from build123d import *

# Parameters (mm, degrees)
SKETCH_1_W      = 50
SKETCH_1_H      = 50
EXTRUDE_1_DEPTH = 2
EXTRUDE_START   = -22.5
SKETCH_3_W      = 13.5
SKETCH_3_H      = 12
SKETCH_3_R      = 1
EXTRUDE_3_DEPTH = 2


with BuildPart() as part:
    # 草图1 → 凸台-拉伸1 (new body)
    with BuildSketch(Plane.XY):
        Rectangle(SKETCH_1_W, SKETCH_1_H)
    extrude(amount=EXTRUDE_1_DEPTH)

    # 草图3 → 凸台-拉伸3 (add)
    with BuildSketch(Plane.XZ.offset(25).offset(EXTRUDE_START)):
        with Locations((-18.25, 8)):
            Rectangle(SKETCH_3_W, SKETCH_3_H)
        with Locations((-13.75, 8)):
            Circle(SKETCH_3_R, mode=Mode.SUBTRACT)
    extrude_3 = extrude(amount=-EXTRUDE_3_DEPTH)

    # 镜向1: 凸台-拉伸3 across plane
    add(extrude_3.mirror(Plane(origin=(0, 0, 0), x_dir=(0, 0, 1), z_dir=(1, 0, 0))))


solid = part.part
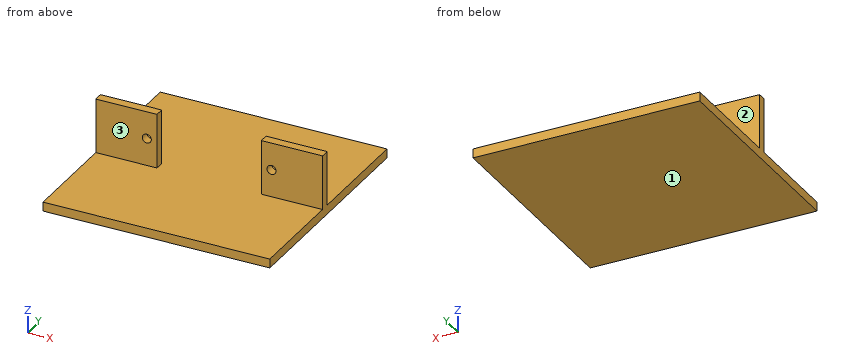
Model file for the job. Use its own axes, mm. Face numbers are marked on the shaded views. A direction names the side the tool comes from. Give positions to 0.01 mm unless a question says otherwise; leave off trailing zeros. Order: outer loops, then holes, each group sorted by start corner. A loop starts at its lowest first (then second) coordinate and runs counter-clockwise, first axis right, second up. Notation, with made-up numbers: (-32, 9.5) - (21, 9.5) arc R9 ccw to (21, 23.5) - close; hole circle Ø1 at (20, 23). An arc over 180 degrees is marked (long way). Write item = value, one per line. Start each with the question number.
1. Which spindle directions (+Z, -Z, +X, -X, +Y, -Y) get a long thin tool onto all of the face, cutting with end or side? Do the marked faces 1, 2 and 3. Say none if no direction does.
2. Probe line 1 along Z through (x, y) = (-13.75, -2.1); line 2 along Y through (x, z) = (15.5, 11); line 3 along Z through (x, y) = (20, 4.5). List the from-to ranges inside material, lowest first.
3. Cut at A-A, the plane z = 12. List the corners of the cut face in (x, y).
4. Cut at C-C, the plane z = 8. List the corners of the cut face in (x, y).
5. Cut at D-D, the plane x = 21.5. List the corners of the cut face in (y, z).
6. Drop flat-ended pins along their axis: P1, Ø2.5, axis at x = -13.75, z = 8, coming from the +Y side; P2, Ø10, axis at x = 6, y = -10, coming from the -Z side; P3, Ø5, axis at x = 17.5, y = -9, coming from the +Z side; P4, Ø1.6, axis at x = 13.75, z = 8, coming from the +Y side. Give the stop position or say it passes through.
7. Cut at B-B, the plane x = 13.75. List the corners of the cut face in (y, z).
Taken from the geometry:
q1.face_1 = -Z, +X, -X, +Y, -Y
q1.face_2 = +Z, +X, -X, +Y
q1.face_3 = +Z, +X, -X, -Y
q2.line_1 = 0 to 7, 9 to 14
q2.line_2 = -2.5 to -0.5
q2.line_3 = 0 to 2
q3.outline = (-25, -2.5) - (-11.5, -2.5) - (-11.5, -0.5) - (-25, -0.5) - close; (11.5, -2.5) - (25, -2.5) - (25, -0.5) - (11.5, -0.5) - close
q4.outline = (-25, -2.5) - (-14.75, -2.5) - (-14.75, -0.5) - (-25, -0.5) - close; (-12.75, -2.5) - (-11.5, -2.5) - (-11.5, -0.5) - (-12.75, -0.5) - close; (11.5, -2.5) - (12.75, -2.5) - (12.75, -0.5) - (11.5, -0.5) - close; (14.75, -2.5) - (25, -2.5) - (25, -0.5) - (14.75, -0.5) - close
q5.outline = (-25, 0) - (25, 0) - (25, 2) - (-0.5, 2) - (-0.5, 14) - (-2.5, 14) - (-2.5, 2) - (-25, 2) - close
q6.P1 = -0.5
q6.P2 = 0
q6.P3 = 2
q6.P4 = through
q7.outline = (-25, 0) - (25, 0) - (25, 2) - (-0.5, 2) - (-0.5, 7) - (-2.5, 7) - (-2.5, 2) - (-25, 2) - close; (-2.5, 9) - (-0.5, 9) - (-0.5, 14) - (-2.5, 14) - close
